```python
from build123d import *

# Parameters (mm, degrees)
SKETCH220_R     = 8
SKETCH220_R_2   = 1.8
PAD127056_DEPTH = 3
SKETCH185_R     = 1.5
PAD127021_DEPTH = 1.75
SKETCH184_W     = 22
SKETCH184_H     = 12
PAD127020_DEPTH = 22.5
PAD127023_DEPTH = 5


with BuildPart() as base:
    # Sketch220 → Pad127056 (new body)
    with BuildSketch(Plane(origin=(50, 160, -8.5), x_dir=(1, 0, 0), z_dir=(0, 0, 1))):
        with BuildLine():
            ThreePointArc((6.010433, -6.010382), (7.852969, 3.252826), (0, 8.5))
            Line((0, 8.5), (-40, 8.5))
            Line((-40, 8.5), (-40, 10.5))
            Line((-40, 10.5), (-43, 10.5))
            Line((-43, 10.5), (-43, 8.5))
            Line((-43, 8.5), (-24.395158, -36.415973))
            Line((-24.395158, -36.415973), (-22.980945, -37.830187))
            Line((-22.980945, -37.830187), (-20.859624, -35.708867))
            Line((-20.859624, -35.708867), (-22.273838, -34.294653))
            Line((6.010433, -6.010382), (-22.273838, -34.294653))
        make_face()
        Circle(SKETCH220_R, mode=Mode.SUBTRACT)
        with Locations((-27, 0)):
            Circle(SKETCH220_R_2, mode=Mode.SUBTRACT)
        with Locations((-27, -10)):
            Circle(SKETCH220_R_2, mode=Mode.SUBTRACT)
        with Locations((-23, -28)):
            Circle(SKETCH220_R_2, mode=Mode.SUBTRACT)
        with Locations((-35, 0)):
            Circle(SKETCH220_R_2, mode=Mode.SUBTRACT)
    extrude(amount=-PAD127056_DEPTH)


with BuildPart() as outerrace:
    # Sketch221 → Revolution010 (revolve)
    with BuildSketch(Plane(origin=(50, 160, -10), x_dir=(1, 0, 0), z_dir=(0, -1, 0))):
        Polygon((5.634953, 1.5), (6.685264, 0), (5.634953, -1.5), (8, -1.5), (8, 1.5), align=None)
    revolve(axis=Axis((50, 160, -10), (0, 0, 1)))


with BuildPart() as pad127021:
    # Sketch185 → Pad127021 (new body)
    with BuildSketch(Plane(origin=(35, 160, 26.5), x_dir=(0, 1, 0), z_dir=(0, 0, 1))):
        Polygon((5.5, 6), (-16.5, 6), (-20.5, 6), (-20.5, -6), (-16.5, -6), (5.5, -6), (9.5, -6), (9.5, 6), align=None)
        with Locations((7.25, 0)):
            Circle(SKETCH185_R, mode=Mode.SUBTRACT)
        with Locations((-18.25, 0)):
            Circle(SKETCH185_R, mode=Mode.SUBTRACT)
    extrude(amount=PAD127021_DEPTH)


with BuildPart() as servovisual:
    # Sketch184 → Pad127020 (new body)
    with BuildSketch(Plane(origin=(35, 160, 11.75), x_dir=(0, 1, 0), z_dir=(0, 0, 1))):
        with Locations((-5.5, 0)):
            Rectangle(SKETCH184_W, SKETCH184_H)
    extrude(amount=PAD127020_DEPTH)

    # Fusion004020023: union Pad127021
    add(pad127021.part)


with BuildPart() as servovisual_1:
    # Fusion004020023 placement: moved
    add(servovisual.part.moved(Location((0, 0, -20))))


with BuildPart() as fusion004020031:
    # Sketch187 → Pad127023 (new body)
    with BuildSketch(Plane(origin=(35, 160, -9), x_dir=(0, 1, 0), z_dir=(0, 0, 1))):
        Polygon((-18, 7.5), (7, 7.5), (7, -6), (-7, -6), (-9, -8), (-16.232233, -8), (-18, -6.232233), align=None)
    extrude(amount=PAD127023_DEPTH)

    # Cut007019029: cut ServoVisual
    add(servovisual_1.part, mode=Mode.SUBTRACT)

    # Fusion004020031: union Base, OuterRace
    add(base.part)
    add(outerrace.part)


with BuildPart() as part_mirroring014:
    # Part__Mirroring014: instance of Fusion004020031
    add(fusion004020031.part.mirror(Plane(origin=(0, 0, 0), x_dir=(0, -1, 0), z_dir=(1, 0, 0))))


solid = part_mirroring014.part
```
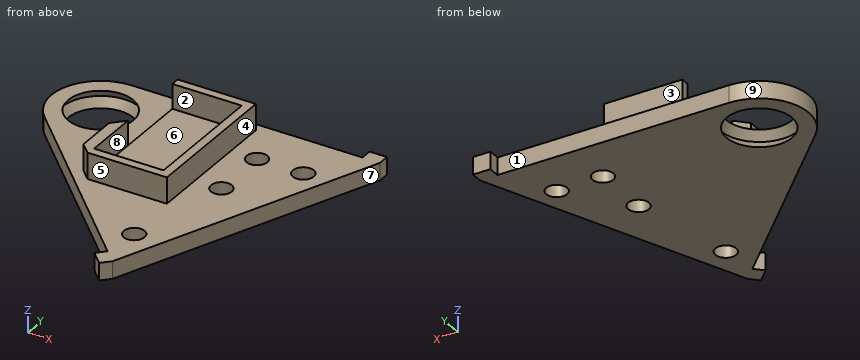
Geometry check sheet. Reference: the model listing, model coordinates, mm. Face numbers are marked on the shaded views. A direction names the side the tool comes from. Coordinates: 2 decimals unless noted, no trailing zeros. Write each loop counter-clockwise with the first axis right and the second up, starting at its lowest first coordinate (ties: lowest second). Pieces come first, ordered by that corner, then holes. Notation, with made-up numbers: M -1.75,2.25 L 45.25,2.25 A28 ccw 45.25,28.25 Z; hole C -22,57.25 d9. An arc over 180 degrees is marked long. One line per item, written item: value. Start each with the question number.
(1) Sectioned sample at B-B, the plane x = -15. Enter the section's corners in (y, z).
(2) Sectioned sample at D-D, the plane x = -23. Enter the section's corners in (y, z).
(3) Tool access check on the marked faces 1, 2, 3, 4 and 5. Record the directions out of +Z, -Z, +X, -X, +Y, -Y that give a thin tool (end or side, any length) a straight path to the whole face; none if there is none.
(4) Depth check by flat-ended pin: pin 1 (5 mm diameter, centred on x = -47.5, y = 164, fed in from +Z); pin 2 (3.5 mm diameter, centred on y = 160.5, z = -5.5, fed in from +X); pin 3 (1.3 mm diameter, centred on x = -35, z = -5, fed in from +Y). Enter the tip coordinate at first touch or a pass-through.
(5) Release check for a two-part mould opening along Y. For the marked faces 6, 7, 8 and 9 record: released by +Y, released by -Y, zero draft, split by the parting line, or undercut.
(6) Sectioned sample at A-A, the plane z = -7.5. Enter the section's corners in (x, y), and give its area (3 significant figures).
(7) Scan lines: line 1 along Y through (x, z) = (-23, -10.3); line 2 along X through (y, z) = (160, -10.7); line 3 along Y through (x, z) = (-15, -9.65). Record each from-to range of solid material in increasing order. Write a range as [from, to].
(8) Sectioned sample at C-C, the plane y = 150. Enter the section's corners in (x, z).
Filled sheet:
1. outline: M 149.19,-11.5 L 158.2,-11.5 L 158.2,-8.5 L 149.19,-8.5 Z; M 161.8,-11.5 L 168.5,-11.5 L 168.5,-8.5 L 161.8,-8.5 Z
2. outline: M 129.87,-11.5 L 148.2,-11.5 L 148.2,-8.5 L 129.87,-8.5 Z; M 151.8,-11.5 L 158.2,-11.5 L 158.2,-8.5 L 151.8,-8.5 Z; M 161.8,-11.5 L 168.5,-11.5 L 168.5,-8.5 L 161.8,-8.5 Z
3. face 1: +Z, -Z, -X, +Y
3. face 2: +Z, -X
3. face 3: +Z, +X, -X, +Y
3. face 4: +Z, +X, +Y, -Y
3. face 5: +Z, +X, -X, -Y
4. pin 1: z = -8.5
4. pin 2: x = -27.5
4. pin 3: y = 167
5. face 6: undercut
5. face 7: released by -Y
5. face 8: undercut
5. face 9: split by the parting line
6. outline: M -43,143.77 L -41.23,142 L -27.5,142 L -27.5,167 L -41,167 L -41,165.5 L -29,165.5 L -29,143.5 L -41,143.5 L -41,153 L -43,151 Z
6. area: 91.9 mm²
7. line 1: [129.87, 148.2], [151.8, 158.2], [161.8, 168.5]
7. line 2: [-58.5, -56.2], [-43.8, -24.8], [-21.2, -16.8], [-13.2, -10.52]
7. line 3: [149.19, 158.2], [161.8, 168.5]
8. outline: M -52.02,-11.5 L -24.8,-11.5 L -24.8,-8.5 L -27.5,-8.5 L -27.5,-4 L -29,-4 L -29,-8.25 L -41,-8.25 L -41,-4 L -43,-4 L -43,-8.5 L -52.02,-8.5 Z; M -21.2,-11.5 L -14.66,-11.5 L -14.66,-8.5 L -21.2,-8.5 Z
